from build123d import *

# Parameters (mm, degrees)
SKETCH_1_R      = 4
EXTRUDE_1_DEPTH = 20


with BuildPart() as part:
    # 草图1 → 凸台-拉伸1 (new body)
    with BuildSketch(Plane(origin=(0, 0, 0), x_dir=(1, 0, 0), z_dir=(0, 1, 0))):
        Polygon((-30, 13.5), (1.5, 13.5), (30, 1.5), (30, -13.5), (-30, -13.5), (-30, -9), (0, -9), (0, 9), (-30, 9), align=None)
        with Locations(Location((10, 1.5, 0), (0, 0, 270))):
            Circle(SKETCH_1_R, mode=Mode.SUBTRACT)
    extrude(amount=EXTRUDE_1_DEPTH)


solid = part.part
The listing builds one solid part. Answer for the finished solid, in the listing's coordinates (mm). A direction names the side the tool comes from. Coordinates: 2 decimals unless noted, no trailing zeros. Order: outer loops, then holes, each group sorted by start corner. A loop starts at its lowest first (then second) coordinate and runs counter-clockwise, first axis right, second up. Notation, with made-up numbers: (62, -10) -> (109, -10) arc R12 ccw to (109, -6) -> close; hole circle Ø8 at (89.5, -25.75). An arc over 180 degrees is marked (long way). Answer in a Markdown table with one row per item. Add a question column.
Item 1: Find section C-C (y = 3.5). Write down the section's boundary in (x, z).
Item 2: Which of the six approach directions +Z, -Z, +X, -X, +Y, -Y give full straight-line access (tool end or side, diameter ignored) to faces 1 (the face through (0, 10, 0)), 2 (the face through (0, 10, 13.5))?
Item 3: Find section B-B (z = 1.5). Write down the section's boundary in (x, y).
Item 4: Determine the mould class of faces 3 (the face through (-14, 10, -13.5)), 4 (the face through (-30, 10, 11)), 5 (the face through (13.966, 9.86, -2.021)) for opening direction X: +X half, -X half, draft (parallel to the pull), parting line (faces both ways), or undercut.
Item 5: Find section D-D (z = 4.5). Write down the section's boundary in (x, y).
Item 6: Find the intervals of material crossed by L1, parallel to Z at x = -22, y = 14; L2, parallel to Z at x = 7.5, y = 7; L3, parallel to X at y = 7.75, z = 6.25, in increasing order. Write a range as from..to.
Item 7: Find section A-A (x = -10). Write down the section's boundary in (y, z).
Item 8: Each of these flat-tipped pins is pushed along its axis until it touches: P1, Ø2, axis at y = 8.5, z = -6.5, coming from the +X side; P2, Ø5, axis at y = 3.5, z = -9.5, coming from the +X side; P3, Ø3, axis at x = 19.5, y = 12.5, coming from the -Z side. Where does it stop, or does it pass through?
Result set:
| question | item | result |
|---|---|---|
| 1 | outline | (-30, -13.5) -> (1.5, -13.5) -> (30, -1.5) -> (30, 13.5) -> (-30, 13.5) -> (-30, 9) -> (0, 9) -> (0, -9) -> (-30, -9) -> close; hole circle Ø8 at (10, -1.5) |
| 2 | face 1 | -X, +Y, -Y |
| 2 | face 2 | +Z, +X, -X, +Y, -Y |
| 3 | outline | (0, 0) -> (7.35, 0) -> (7.35, 20) -> (0, 20) -> close; (12.65, 0) -> (30, 0) -> (30, 20) -> (12.65, 20) -> close |
| 4 | face 3 | draft |
| 4 | face 4 | -X half |
| 4 | face 5 | undercut |
| 5 | outline | (0, 0) -> (30, 0) -> (30, 20) -> (0, 20) -> close |
| 6 | L1 | z = -13.5..-9, 9..13.5 |
| 6 | L2 | z = -10.97..-4.62, 1.62..13.5 |
| 6 | L3 | x = 0..30 |
| 7 | outline | (0, -13.5) -> (20, -13.5) -> (20, -9) -> (0, -9) -> close; (0, 9) -> (20, 9) -> (20, 13.5) -> (0, 13.5) -> close |
| 8 | P1 | stops at x = 20.5 |
| 8 | P2 | stops at x = 16.94 |
| 8 | P3 | stops at z = -6.55 |
